Job drawing, mm, ordinate dimensions from the low corner. One solid piece. A direction names the side the tool comes from. Give positions to 0.01 mm unless a question says otherwise; leave off trailing zeros. Order: outer loops, then holes, each group sorted by start corner. A loop starts at its lowest first (then second) coordinate and runs counter-clockwise, first axis right, second up. Notation, with made-up numbers: M 79.25,-14.5 L 118.25,-14.5 A21 cw 118.25,-6.5 Z; hole C 12.5,-37.75 d1. An arc over 180 degrees is marked long. Use CSV: the item, a comma, the result in double quotes. Start each with the question number.
Item 1: Wall check: line 1 along Z through (x, y) = (38, 7.5); line 2 along Z through (x, y) = (4, 2); line 3 along X through (y, z) = (2.5, 8.25). Give the ranges that are in metal, low to high.
Item 2: Band-saw the part on D-D on y = 1.5. Write the cut outline in (x, z) (3 decimals).
Item 3: Band-saw the part on B-B on x = 11.5. Write the cut outline in (y, z), plus the area to 3 significant figures.
Item 4: Two-plate mould, pull along Z, no slides. Class the marked faces 3, 4 and 5: pulls with the +Z half, pulls with the -Z half, needs draft (parallel to the pull), parting line crosses it, or undercut.
Item 5: Pin check, flat tips, straight feed: P1, Ø3, axis at x = 17, y = 5, coming from the +Z side; P2, Ø8, axis at x = 7.5, z = 6.5, coming from the -Y side; P3, Ø1.5, axis at y = 5.5, z = 6.5, coming from the +X side. Stop position of each tip, or through.
Item 6: Band-saw the part on A-A on y = 7.5. Write the cut outline in (x, z) (3 decimals), plus the area to 3 significant figures.
Item 7: Which spindle directions (+Z, -Z, +X, -X, +Y, -Y) get a long thin tool onto all of the face, cutting with end or side? Do the marked faces 1 and 2. Say none if no direction does.
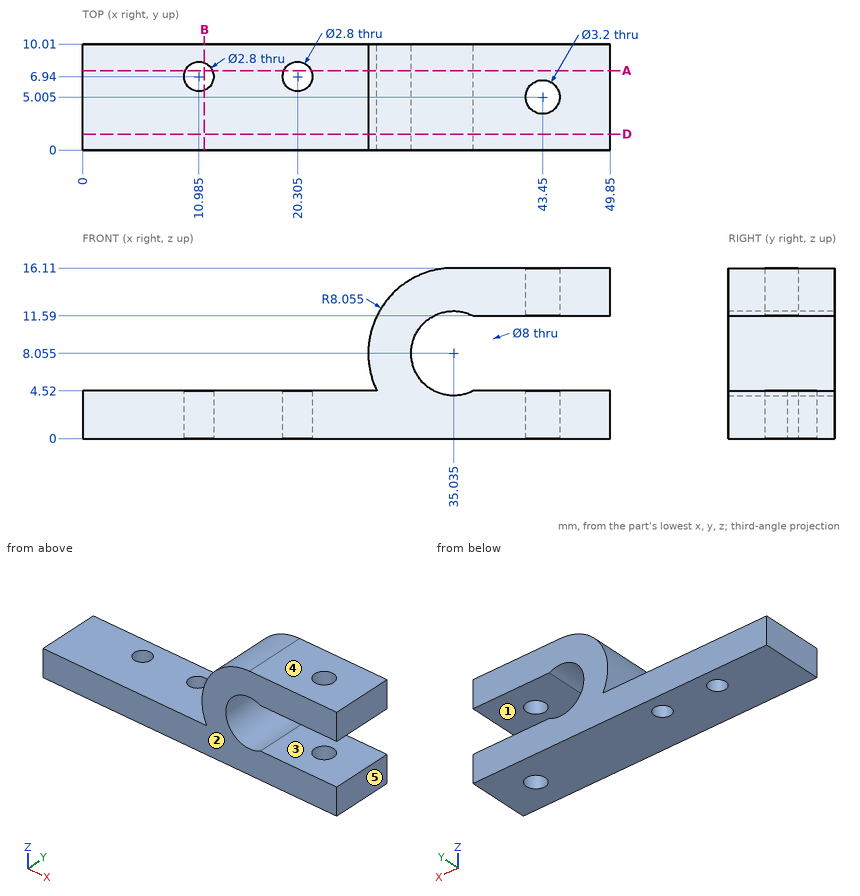
Model answer:
1,line 1,"z = 0 to 4.52, 11.59 to 16.11"
1,line 2,"z = 0 to 4.52"
1,line 3,"x = 26.98 to 31.04"
2,outline,"M 0,0 L 49.85,0 L 49.85,4.52 L 36.907,4.52 A4 cw long 36.907,11.59 L 49.85,11.59 L 49.85,16.11 L 35.035,16.11 A8.055 ccw 27.797,4.52 L 0,4.52 Z"
3,outline,"M 0,0 L 5.64,0 L 5.64,4.52 L 0,4.52 Z; M 8.24,0 L 10.01,0 L 10.01,4.52 L 8.24,4.52 Z"
3,area,"33.5 mm^2"
4,face 3,"undercut"
4,face 4,"pulls with the +Z half"
4,face 5,"needs draft"
5,P1,"stops at z = 4.52"
5,P2,"stops at y = 0"
5,P3,"stops at x = 31.77"
6,outline,"M 0,0 L 9.702,0 L 9.702,4.52 L 0,4.52 Z; M 12.268,0 L 19.022,0 L 19.022,4.52 L 12.268,4.52 Z; M 21.588,0 L 49.85,0 L 49.85,4.52 L 36.907,4.52 A4 cw long 36.907,11.59 L 49.85,11.59 L 49.85,16.11 L 35.035,16.11 A8.055 ccw 27.797,4.52 L 21.588,4.52 Z"
6,area,"321 mm^2"
7,face 1,"+X, +Y, -Y"
7,face 2,"+Z, -Z, +X, -X, -Y"
